Check sheet for the modelled part. Datum: model origin and axes. Units: mm. Face numbers are marked on the shaded views. A direction names the side the tool comes from. Give positions to 0.01 mm unless a question says otherwise; leave off trailing zeros. Loops run counter-clockwise (first coordinate to the right, second up) from the corner with the lowest first, then second, coordinate; pieces in that order, holes last. Notation, with made-up numbers: (-15, 57.25) - (9, 57.25) arc R28 cw to (9, 93.25) - close; hole circle Ø4 at (64, -15). An arc over 180 degrees is marked (long way). Use one line per item in the form item = value.
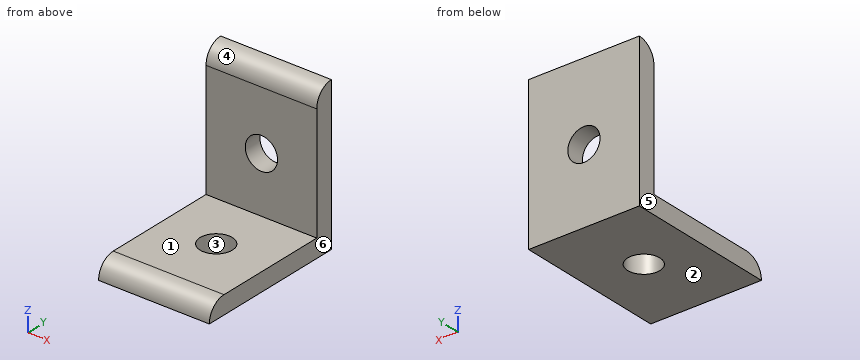
from build123d import *

# Parameters (mm, degrees)
ESBO_O1_W                = 18.22
ESBO_O1_H                = 25
RESSALTO_EXTRUS_O1_DEPTH = 3
ESBO_O2_W                = 18.22
ESBO_O2_H                = 3
RESSALTO_EXTRUS_O2_DEPTH = 22
ESBO_O3_R                = 2.65
CORTE_EXTRUS_O1_DEPTH    = 25
ESBO_O4_R                = 2.65
CORTE_EXTRUS_O2_DEPTH    = 25
FILETE1_R                = 3


with BuildPart() as part:
    # Esboço1 → Ressalto-extrusão1 (new body)
    with BuildSketch(Plane.XY):
        with Locations((-79.470886401, -322.165681156)):
            Rectangle(ESBO_O1_W, ESBO_O1_H)
    extrude(amount=RESSALTO_EXTRUS_O1_DEPTH)

    # Esboço2 → Ressalto-extrusão2 (add)
    with BuildSketch(Plane.XY.offset(3)):
        with Locations((-79.470886401, -311.165681156)):
            Rectangle(ESBO_O2_W, ESBO_O2_H)
    extrude(amount=RESSALTO_EXTRUS_O2_DEPTH)

    # Esboço3 → Corte-extrusão1 (cut)
    with BuildSketch(Plane.XY.offset(3)):
        with Locations((-79.470886401, -321.915681156)):
            Circle(ESBO_O3_R)
    extrude(amount=-CORTE_EXTRUS_O1_DEPTH, mode=Mode.SUBTRACT)

    # Esboço4 → Corte-extrusão2 (cut)
    with BuildSketch(Plane.XZ.offset(312.665681156)):
        with Locations(Location((-79.470886401, 12.25, 0), (0, 0, 270))):
            Circle(ESBO_O4_R)
    extrude(amount=-CORTE_EXTRUS_O2_DEPTH, mode=Mode.SUBTRACT)

    # Filete1
    filete1_edges = [part.edges().sort_by_distance(p)[0] for p in [
        (-79.470886401, -312.665681156, 25),
        (-79.470886401, -334.665681156, 3),
    ]]
    fillet(filete1_edges, radius=FILETE1_R - 0.0001)  # a hair under: the kernel refuses the full size


solid = part.part
Item 1: Section check C-C on y = -322.25. Record the boundary of the cut face in (x, z).
Answer block:
outline = (-88.58, 0) - (-82.1, 0) - (-82.1, 3) - (-88.58, 3) - close; (-76.84, 0) - (-70.36, 0) - (-70.36, 3) - (-76.84, 3) - close
Item 2: Mould release check, pull along X, two halves, no side actions. Record for the marked faces 3, 4, 5 and 6: released by +X, released by -X, zero draft, split by the parting line, or undercut.
Answer block:
face_3 = undercut
face_4 = zero draft
face_5 = released by -X
face_6 = released by +X
Item 3: Access from +Z, -Z, +X, -X, +Y, -Y to the whole of each face (thin tool, end or side, straight path). Record for the marked faces 1 and 2.
Answer block:
face_1 = +Z, +X, -X, -Y
face_2 = -Z, +X, -X, +Y, -Y
Item 4: Section check B-B on x = -77.5. Give the number of separate pieces and of enclosed holes in the cut face, then the cut area to 3 significant figures.
Answer block:
separate_pieces = 3
enclosed_holes = 0
area = 116 mm2
Item 5: Thickness scan on L1, parallel to X at y = -311.1, z = 12.25; L2, parallel to Y at x = -78.25, z = 3.75; L3, parallel to Z at x = -83.5, y = -326.5. Record the ranges inside material, lowest first.
Answer block:
L1 = -88.58 to -82.12, -76.82 to -70.36
L2 = -312.67 to -309.67
L3 = 0 to 3
Item 6: Section check A-A on z = 12.25. Record the boundary of the cut face in (x, y), then the cut area to 3 significant figures.
Answer block:
outline = (-88.58, -312.67) - (-82.12, -312.67) - (-82.12, -309.67) - (-88.58, -309.67) - close; (-76.82, -312.67) - (-70.36, -312.67) - (-70.36, -309.67) - (-76.82, -309.67) - close
area = 38.8 mm2
Item 7: Section check D-D on z = 16.5. Record the boundary of the cut face in (x, y), then the cut area to 3 significant figures.
Answer block:
outline = (-88.58, -312.67) - (-70.36, -312.67) - (-70.36, -309.67) - (-88.58, -309.67) - close
area = 54.7 mm2
Item 8: Gauge pin test, flat ends, axial feed: P1, Ø6, axis at y = -319, z = 7.5, coming from the -X side; P2, Ø5.5, axis at x = -80.5, z = 16.5, coming from the -Y side; P3, Ø9, axis at x = -83.5, y = -320, coming from the +Z side; P4, Ø6, axis at x = -77.5, y = -314, coming from the +Z side. Record the tip position at first contact, or that the pin passes through.
Answer block:
P1 = through
P2 = -312.67
P3 = 3
P4 = 24.69
